Geometry: final body of the model. Coordinates: model frame, mm. Coordinates: 2 decimals unless noted, no trailing zeros. Write each loop counter-clockwise with the first axis right and the second up, starting at its lowest first coordinate (ties: lowest second). Pieces come first, ordered by that corner, then holes. Notation, with made-up numbers: (53, 17.25) -> (95, 17.25) arc R16 cw to (95, 25.25) -> close; hole circle Ø8 at (48, 63). An arc over 180 degrees is marked (long way). One line per item, written item: value.
Autodesk Fusion 360 part; units mm, degrees
sketch "Sketch1" plane through (0, 0, 0) normal (0, 0, 1) x (1, 0, 0) in component "TR8x2_Nut"
  line L0 (17, 16.5) -> (-17, 16.5)
  line L1 (-17, 16.5) -> (-17, -16.5)
  line L2 (-17, -16.5) -> (17, -16.5)
  line L3 (17, -16.5) -> (17, 16.5)
  line L4 (17, 16.5) -> (-17, -16.5) construction
  line L5 (-17, 16.5) -> (17, -16.5) construction
  line L6 (-9, -8.5) -> (17, -8.5)
  line L7 (-9, -3.5) -> (17, -3.5)
  line L8 (-17, 6.5) -> (17, 6.5) construction
  line L9 (-9, -8.5) -> (-9, -3.5) construction
  arc A0 (-9, -3.5) -> (-9, -8.5) centre (-9, -6) ccw
  circle A1 centre (-10, 6.5) radius 2.55
  line L10 (0, 0) -> (0, 16.5) construction
  circle A2 centre (10, 6.5) radius 2.55
  dimension "d1" = 34
  dimension "d2" = 33
  dimension "d7" = 26
  dimension "d8" = 5.1
  dimension "d9" = 7
  dimension "d10" = 10
  dimension "d11" = 20
  dimension "d12" = 5
extrude "Extrude1" add sketch "Sketch1" along normal mid plane 12 contours L0 L1 L2 L3 L6 L7 A0 in component "TR8x2_Nut"
sketch "Sketch2" plane through (0, 0, 0) normal (0, 1, 0) x (1, 0, 0) in component "TR8x2_Nut"
  circle A0 centre (0, 0) radius 4
  circle A1 centre (10, 0) radius 2.5
  dimension "d15" = 8
  dimension "d16" = 5
  dimension "d17" = 10
extrude "Extrude2" cut sketch "Sketch2" against normal blind 12.9576 from surface at -8.5 contours A1 in component "TR8x2_Nut"
extrude "Extrude3" cut sketch "Sketch2" along normal mid plane 84.5817 contours A0 in component "TR8x2_Nut"
fillet "Fillet1" radius 3 4 edges at (-17, -16.5, 0) (17, -16.5, 0) (17, 16.5, 0) (-17, 16.5, 0) in component "TR8x2_Nut"
component "TR8x2_Nut" placed x (1, 0, 0) y (0, 1, 0) z (0, 0, 1) at (0, 0, 0)
(1) Line query: line 1 (Z direction, x = 10, y = -12.5); line 2 (Z direction, x = 0, y = -12.5); line 3 (Y direction, x = -10, z = -0.5). Output: solid intervals per line, ascending. Write a range as [from, to].
Responses:
line 1: z = [-6, -2.5], [2.5, 6]
line 2: z = [-6, -4], [4, 6]
line 3: y = [-16.5, -8.29], [-3.71, 3.95], [9.05, 16.5]
(2) Section B-B (z = -1.75). Return the cut outline in (x, y), then the cut area to 3 significant figures.
Responses:
outline: (-17, -13.5) arc R3 ccw to (-14, -16.5) -> (-3.6, -16.5) -> (-3.6, -8.5) -> (-9, -8.5) arc R2.5 cw to (-9, -3.5) -> (-3.6, -3.5) -> (-3.6, 16.5) -> (-14, 16.5) arc R3 ccw to (-17, 13.5) -> close; (3.6, -16.5) -> (8.21, -16.5) -> (8.21, -8.5) -> (3.6, -8.5) -> close; (3.6, -3.5) -> (17, -3.5) -> (17, 13.5) arc R3 ccw to (14, 16.5) -> (3.6, 16.5) -> close; (11.79, -16.5) -> (14, -16.5) arc R3 ccw to (17, -13.5) -> (17, -8.5) -> (11.79, -8.5) -> close; hole circle Ø5.1 at (-10, 6.5); hole circle Ø5.1 at (10, 6.5)
area: 704 mm2
(3) Section D-D (x = -12). Return the cut outline in (y, z), then the cut area to 3 significant figures.
Responses:
outline: (-16.5, -6) -> (4.92, -6) -> (4.92, 6) -> (-16.5, 6) -> close; (8.08, -6) -> (16.5, -6) -> (16.5, 6) -> (8.08, 6) -> close
area: 358 mm2
(4) Section C-C (y = 5.5). Return the cut outline in (x, z).
Responses:
outline: (-17, -6) -> (-12.35, -6) -> (-12.35, 6) -> (-17, 6) -> close; (-7.65, -6) -> (7.65, -6) -> (7.65, 6) -> (-7.65, 6) -> close; (12.35, -6) -> (17, -6) -> (17, 6) -> (12.35, 6) -> close; hole circle Ø8 at (0, 0)
(5) Section A-A (x = 10). Return the cut outline in (y, z).
Responses:
outline: (-16.5, -6) -> (-8.5, -6) -> (-8.5, -2.5) -> (-16.5, -2.5) -> close; (-16.5, 2.5) -> (-8.5, 2.5) -> (-8.5, 6) -> (-16.5, 6) -> close; (-3.5, -6) -> (3.95, -6) -> (3.95, 6) -> (-3.5, 6) -> close; (9.05, -6) -> (16.5, -6) -> (16.5, 6) -> (9.05, 6) -> close
(6) Pull-direction query (Z, two-part tool) for faces 1 (the cylindrical face through (-0.867, 6.64, 3.905)), 2 (the cylindrical face through (7.5, -12.4, -0.1)), 3 (the flat face through (7, -8.5, 0)), 4 (the flat face through (0, 0, -6)); classes: released by +Z, released by -Z, zero draft, split by the parting line, or undercut.
Responses:
face 1: undercut
face 2: undercut
face 3: zero draft
face 4: released by -Z
